Autodesk Inventor part; units mm, degrees
ref_plane "YZ Plane" through (0, 0, 0) normal (1, 0, 0) x (0, 1, 0)
ref_plane "XZ Plane" through (0, 0, 0) normal (0, 1, 0) x (-1, 0, 0)
ref_plane "XY Plane" through (0, 0, 0) normal (0, 0, 1) x (1, 0, 0)
ref_plane "Work Plane1" through (0, -0.0041, 0) normal (0, 0, 1) x (1, 0, 0)
sketch "Sketch1" plane through (0, -0.0041, 0) normal (0, 0, 1) x (1, 0, 0)
  line L0 (0, -194.9959) -> (0, 0.0041) construction
  line L1 (9, 0.0041) -> (9, -194.9959) construction
  circle A0 centre (4.5, -53.479) radius 1.7 construction
  circle A1 centre (4.5, -33.921) radius 1.7 construction
  circle A2 centre (4.5, -53.479) radius 1.7
  circle A3 centre (4.5, -33.921) radius 1.7
  line L2 (4.5, -53.479) -> (4.5, -59.829) construction
  line L3 (4.5, -33.921) -> (4.5, -27.571) construction
  line L4 (9, -27.5751) -> (0, -27.5751)
  line L5 (4.5, -59.829) -> (9, -59.829)
  line L6 (9, -27.5751) -> (9, -59.829)
  line L7 (4.5, -59.829) -> (0, -59.829)
  line L8 (0, -27.5751) -> (0, -59.829)
  dimension "d0" = 6.35
  dimension "d1" = 6.35
extrude "Extrusion1" add sketch "Sketch1" along normal blind 1.524
properties part number "standoff for gripper servo"
Part model, mm, in its own coordinate system. Round coordinates to 2 decimals unless told otherwise and drop trailing zeros. Loops run counter-clockwise (first coordinate to the right, second up) from the corner with the lowest first, then second, coordinate; pieces in that order, holes last.
Item 1: Mould opens along X. For faces 1 (the face through (4, -59.833, 1)), 2 (the face through (4.28, -55.17, 0.75)), 3 (the face through (9, -43, 1)) say: +X half, -X half, draft (parallel to the pull), parting line (faces both ways), or undercut.
Item 2: Cut at B-B, the plane z = 0.85. Give the cut face in (x, y).
Item 3: Cut at A-A, the plane x = 4.5. Give the cut face in (y, z).
Item 4: Drill centre lines: line 1 (Y direction, x = 4.5, z = 1.1); line 2 (X direction, y = -34, z = 0.8); line 3 (Y direction, x = 5, z = 0.7). Where is each one in solid material? Low to high.
Item 5: Drop a flat-ended pin along its axis: P1, Ø4.5, axis at x = 4.5, y = -33.93, coming from the -Z side. Give the stop position or say it passes through.
A:
1. face 1: draft
1. face 2: undercut
1. face 3: +X half
2. outline: (0, -59.83) - (9, -59.83) - (9, -27.58) - (0, -27.58) - close; hole circle Ø3.4 at (4.5, -53.48); hole circle Ø3.4 at (4.5, -33.93)
3. outline: (-59.83, 0) - (-55.18, 0) - (-55.18, 1.52) - (-59.83, 1.52) - close; (-51.78, 0) - (-35.63, 0) - (-35.63, 1.52) - (-51.78, 1.52) - close; (-32.23, 0) - (-27.58, 0) - (-27.58, 1.52) - (-32.23, 1.52) - close
4. line 1: y = -59.83 to -55.18, -51.78 to -35.63, -32.23 to -27.58
4. line 2: x = 0 to 2.8, 6.2 to 9
4. line 3: y = -59.83 to -55.11, -51.86 to -35.55, -32.3 to -27.58
5. P1: stops at z = 0
